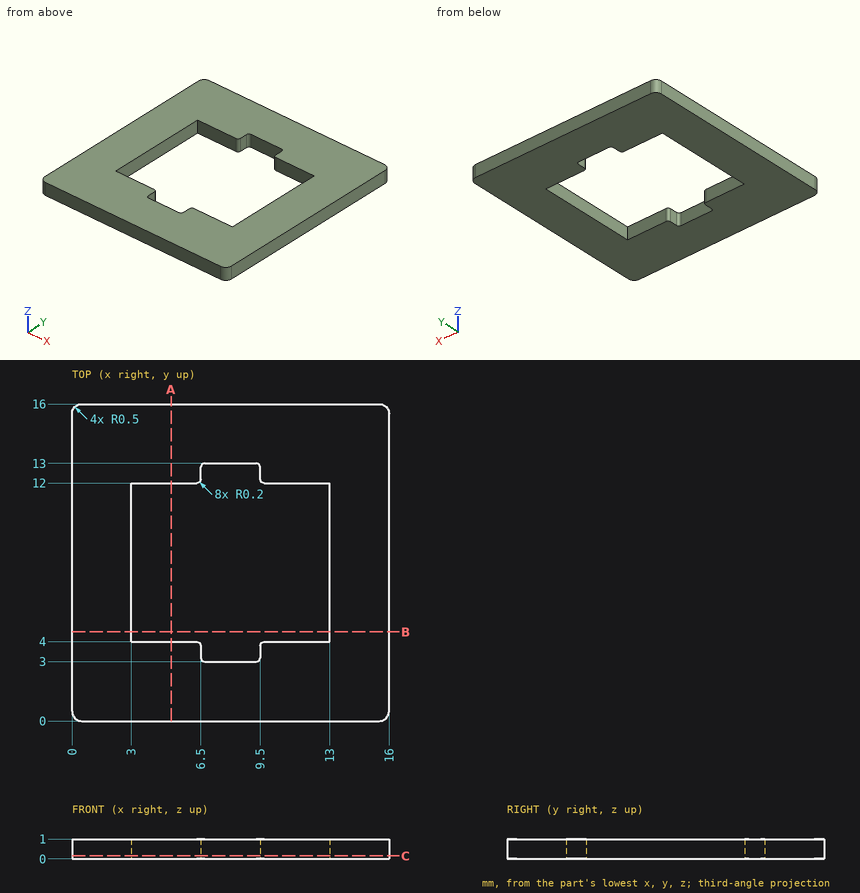
The drawing under review shows one solid part. Ordinate dimensions are in mm from its lowest x, y, z. Round coordinates to 2 decimals unless told otherwise and drop trailing zeros. Write each loop counter-clockwise with the first axis right and the second up, starting at its lowest first coordinate (ties: lowest second). Pieces come first, ordered by that corner, then holes. Notation, with made-up numbers: (23.5, 69) -> (68.5, 69) arc R22 ccw to (68.5, 98) -> close; hole circle Ø7 at (-10.5, 17). An arc over 180 degrees is marked (long way). One line per question, with ' | ' between items.
(1) Take a section at A-A, the plane x = 5. State the section outline as (y, z) points, and give its area (3 significant figures).
Result sheet:
outline: (0, 0) -> (4, 0) -> (4, 1) -> (0, 1) -> close; (12, 0) -> (16, 0) -> (16, 1) -> (12, 1) -> close | area: 8.00 mm2
(2) Take a section at B-B, the plane y = 4.5. State the section outline as (x, z) points.
Result sheet:
outline: (0, 0) -> (3, 0) -> (3, 1) -> (0, 1) -> close; (13, 0) -> (16, 0) -> (16, 1) -> (13, 1) -> close
(3) Wall thickness on line 1 (X direction, y = 9.75, z = 0.9); line 2 (Y direction, x = 12.5, z = 0.2): over which ranges is each line inside the solid? List them lowest first. Write a range as [from, to].
Result sheet:
line 1: [0, 3], [13, 16] | line 2: [0, 4], [12, 16]
(4) Take a section at C-C, the plane z = 0.15. State the section outline as (x, y) points.
Result sheet:
outline: (0, 0.5) arc R0.5 ccw to (0.5, 0) -> (15.5, 0) arc R0.5 ccw to (16, 0.5) -> (16, 15.5) arc R0.5 ccw to (15.5, 16) -> (0.5, 16) arc R0.5 ccw to (0, 15.5) -> close; hole (3, 4) -> (6.3, 4) arc R0.2 cw to (6.5, 3.8) -> (6.5, 3.2) arc R0.2 ccw to (6.7, 3) -> (9.3, 3) arc R0.2 ccw to (9.5, 3.2) -> (9.5, 3.8) arc R0.2 cw to (9.7, 4) -> (13, 4) -> (13, 12) -> (9.7, 12) arc R0.2 cw to (9.5, 12.2) -> (9.5, 12.8) arc R0.2 ccw to (9.3, 13) -> (6.7, 13) arc R0.2 ccw to (6.5, 12.8) -> (6.5, 12.2) arc R0.2 cw to (6.3, 12) -> (3, 12) -> close
